```python
from build123d import *

# Parameters (mm, degrees)
SKETCH1_W   = 10
SKETCH1_H   = 60
SKETCH1_W_2 = 0.1
SKETCH1_H_2 = 20


with BuildPart() as part:
    # Sketch1 → Revolve1 (revolve)
    with BuildSketch(Plane.XY, mode=Mode.PRIVATE) as revolve1_sk:
        with Locations((10, 30)):
            Rectangle(SKETCH1_W, SKETCH1_H)
        with Locations((15.05, 45)):
            Rectangle(SKETCH1_W_2, SKETCH1_H_2)
        with Locations((15.05, 10)):
            Rectangle(SKETCH1_W_2, SKETCH1_H_2)
    revolve(revolve1_sk.sketch.rotate(Axis((0, 0, 0), (0, 1, 0)), 90), axis=Axis((0, 0, 0), (0, 1, 0)))


solid = part.part
```
CAD build for the part. Positions are in the model's coordinates, mm. A direction names the side the tool comes from. Give positions to 0.01 mm unless a question says otherwise; leave off trailing zeros. Order: outer loops, then holes, each group sorted by start corner. A loop starts at its lowest first (then second) coordinate and runs counter-clockwise, first axis right, second up.
(1) Saw through at B-B, the plane z = 0. Give the cut face in (x, y).
(2) Mould opens along Z. For faces 3 (the cylindrical face through (-12.65, 57.54, -8.06)), 4 (the cylindrical face through (0, 30, 5)), 5 (the flat face through (-4, 0, -4)) say: released by +Z, released by -Z, zero draft, split by the parting line, or undercut.
(3) Saw through at C-C, the plane y = 13. Give the cut face in (x, z), then the cut area to 3 significant figures.
(4) Saw through at A-A, the plane x = 0. Give the cut face in (y, z), then the cut area to 3 significant figures.
(5) Saw through at D-D, the plane x = -11. Give the cut face in (y, z), then the cut area to 3 significant figures.
(6) Flat gauge pins, fed straight in: pin 1 (3 mm diameter, centred on x = -6.5, y = 52, fed in from +Z); pin 2 (9 mm diameter, centred on x = -6, z = 5, fed in from -Y); pin 3 (1.5 mm diameter, centred on y = 25.5, z = -11, fed in from +X); pin 4 (2 mm diameter, centred on x = 10, y = 46.5, fed in from -Z). Where does each tip first touch, or does it go through?
(7) Drill centre lines: L1, parallel to X at y = 46, z = 0; L2, parallel to X at y = 22, z = 0; L3, parallel to Z at x = 2, y = 6.5. Where is each one in solid material? Low to high.
(8) Tool access for faces 1 (the flat face through (-4, 60, -4)), 2 (the cylindrical face through (-12.65, 27.6, -8.06)): list every direction of +Z, -Z, +X, -X, +Y, -Y with a clear straight run to the whole face (end or side of a thin tool).
Results found:
1. outline: (-15.1, 0) - (-5, 0) - (-5, 60) - (-15, 60) - (-15, 55) - (-15.1, 55) - (-15.1, 35) - (-15, 35) - (-15, 20) - (-15.1, 20) - close; (5, 0) - (15.1, 0) - (15.1, 20) - (15, 20) - (15, 35) - (15.1, 35) - (15.1, 55) - (15, 55) - (15, 60) - (5, 60) - close
2. face 3: split by the parting line
2. face 4: undercut
2. face 5: zero draft
3. outline: circle Ø30.2 at (0, 0); hole circle Ø10 at (0, 0)
3. area: 638 mm2
4. outline: (0, -15.1) - (20, -15.1) - (20, -15) - (35, -15) - (35, -15.1) - (55, -15.1) - (55, -15) - (60, -15) - (60, -5) - (0, -5) - close; (0, 5) - (60, 5) - (60, 15) - (55, 15) - (55, 15.1) - (35, 15.1) - (35, 15) - (20, 15) - (20, 15.1) - (0, 15.1) - close
4. area: 1,210 mm2
5. outline: (0, -10.34) - (20, -10.34) - (20, -10.2) - (35, -10.2) - (35, -10.34) - (55, -10.34) - (55, -10.2) - (60, -10.2) - (60, 10.2) - (55, 10.2) - (55, 10.34) - (35, 10.34) - (35, 10.2) - (20, 10.2) - (20, 10.34) - (0, 10.34) - close
5. area: 1,240 mm2
6. pin 1: stops at z = 14.25
6. pin 2: stops at y = 0
6. pin 3: stops at x = 10.95
6. pin 4: stops at z = -12.12
7. L1: x = -15.1 to -5, 5 to 15.1
7. L2: x = -15 to -5, 5 to 15
7. L3: z = -14.97 to -4.58, 4.58 to 14.97
8. face 1: +Z, -Z, +X, -X, +Y
8. face 2: none
